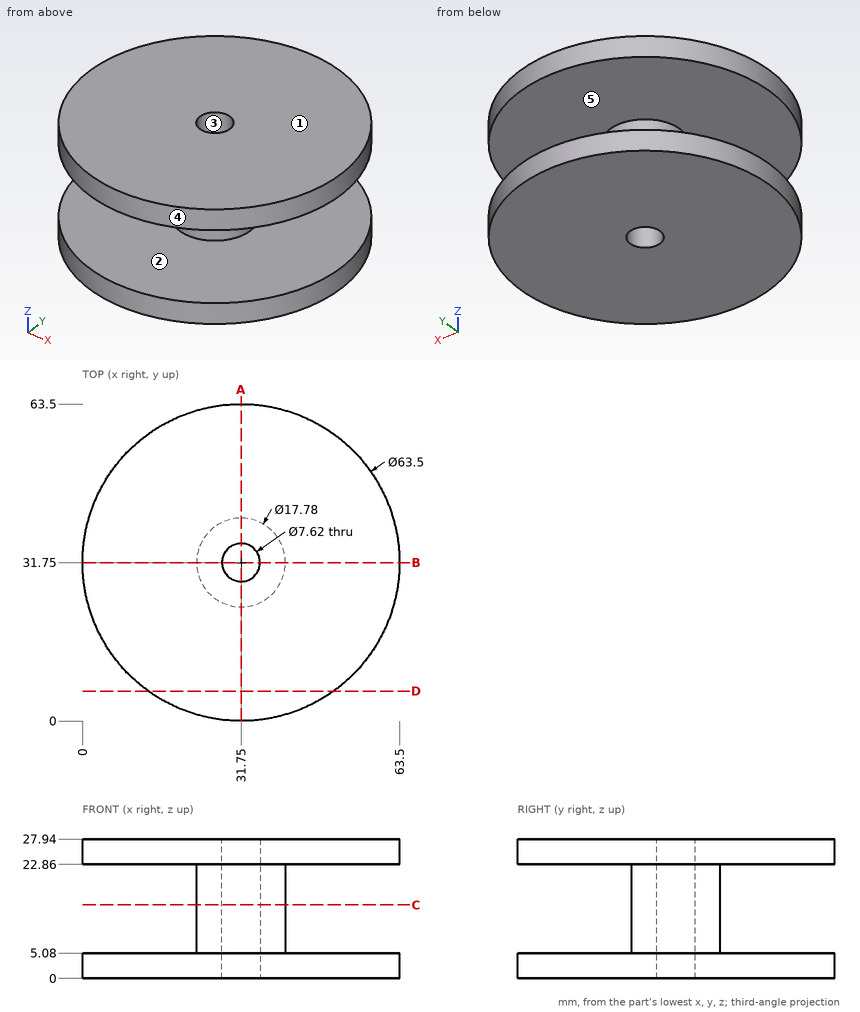
Geometry: see drawing. Coordinates: mm, zero at the bounding-box minimum. A direction names the side the tool comes from. Give positions to 0.01 mm unless a question says otherwise; leave off trailing zeros. Loops run counter-clockwise (first coordinate to the right, second up) from the corner with the lowest first, then second, coordinate; pieces in that order, holes last. Notation, with made-up numbers: (77.5, 50.5) -> (89.5, 50.5) arc R24 ccw to (89.5, 75.5) -> close; hole circle Ø9 at (42, 0.25). An arc over 180 degrees is marked (long way). Put each result on its own line as item: value.
1. Pull-direction query (Z, two-part tool) for the marked faces 1, 2 and 3; classes: released by +Z, released by -Z, zero draft, split by the parting line, or undercut.
Taken from the geometry:
face 1: released by +Z
face 2: undercut
face 3: zero draft
2. Cut plane D-D (y = 6). Return the cut outline in (x, z), plus the area to 3 significant figures.
Taken from the geometry:
outline: (13.18, 0) -> (50.32, 0) -> (50.32, 5.08) -> (13.18, 5.08) -> close; (13.18, 22.86) -> (50.32, 22.86) -> (50.32, 27.94) -> (13.18, 27.94) -> close
area: 377 mm2
3. Cut plane A-A (x = 31.75). Return the cut outline in (y, z).
Taken from the geometry:
outline: (0, 0) -> (27.94, 0) -> (27.94, 27.94) -> (0, 27.94) -> (0, 22.86) -> (22.86, 22.86) -> (22.86, 5.08) -> (0, 5.08) -> close; (35.56, 0) -> (63.5, 0) -> (63.5, 5.08) -> (40.64, 5.08) -> (40.64, 22.86) -> (63.5, 22.86) -> (63.5, 27.94) -> (35.56, 27.94) -> close
4. Ray query, line 1 along Z through (x, y) = (25.5, 44); line 2 along Y through (x, z) = (32, 25.25); line 3 along Y through (x, z) = (31.75, 19.75). Return the intervals inside material, ascending. Write a range as [from, to].
Taken from the geometry:
line 1: z = [0, 5.08], [22.86, 27.94]
line 2: y = [0, 27.95], [35.55, 63.5]
line 3: y = [22.86, 27.94], [35.56, 40.64]
5. Set-up query: the marked faces 4 and 5. Return all of +Z, -Z, +X, -X, +Y, -Y with unobstructed straight access to the full face (end or side cutting, diameter ignored); none if empty.
Taken from the geometry:
face 4: +Z, -Z
face 5: none
6. Cut plane C-C (z = 14.75). Return the cut outline in (x, y), plus the area to 3 significant figures.
Taken from the geometry:
outline: circle Ø17.78 at (31.75, 31.75); hole circle Ø7.62 at (31.75, 31.75)
area: 203 mm2
